Input: dimensioned drawing with shaded views. Units: mm. Origin: part minimum x, y, z. Give positions to 0.01 mm unless a question says otherwise; leave off trailing zeros. Order: outer loops, then holes, each group sorted by start corner. A loop starts at its lowest first (then second) coordinate and runs counter-clockwise, first axis right, second up. Notation, with made-up numbers: (35, 43.25) -> (43, 43.25) arc R35 ccw to (43, 80.25) -> close; hole circle Ø6 at (48, 19.25). An arc over 180 degrees is marked (long way). Use CSV: the item, a comma, the result in double quotes.
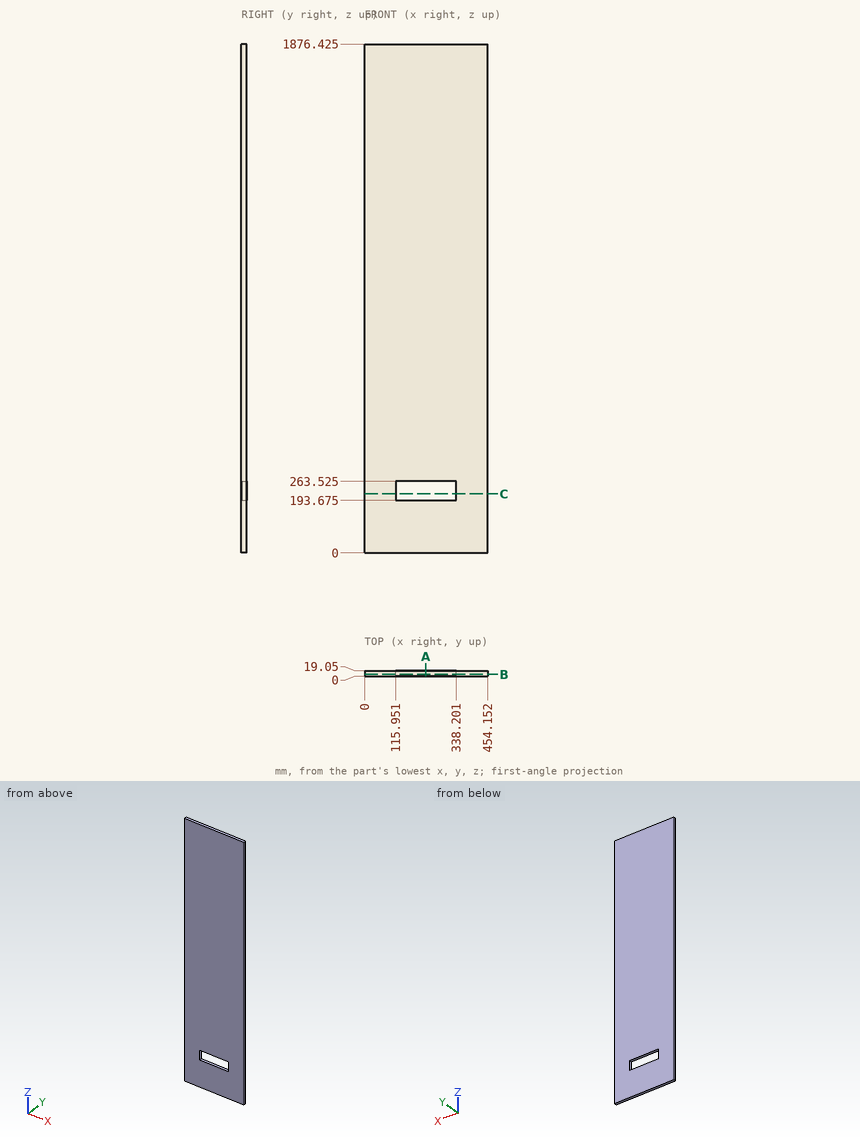
1. Section query A-A on x = 226.5. Return loops of the section in (y, z) (3 decimals), plus the area to 3 significant figures.
Answer below:
outline,"(0, 0) -> (19.05, 0) -> (19.05, 193.675) -> (0, 193.675) -> close; (0, 263.525) -> (19.05, 263.525) -> (19.05, 1876.425) -> (0, 1876.425) -> close"
area,"34,400 mm²"
2. Section query B-B on y = 6. Return loops of the section in (x, z) (3 decimals).
Answer below:
outline,"(0, 0) -> (454.152, 0) -> (454.152, 1876.425) -> (0, 1876.425) -> close; hole (115.951, 193.675) -> (338.201, 193.675) -> (338.201, 263.525) -> (115.951, 263.525) -> close"
3. Ray query, line 1 along Z through (x, y) = (288, 9) (3 decimals). Return the intervals inside material, ascending.
Answer below:
line 1,"z = 0 to 193.675, 263.525 to 1876.425"
4. Section query C-C on z = 217. Return loops of the section in (x, y), plus the area to 3 significant figures.
Answer below:
outline,"(0, 0) -> (115.95, 0) -> (115.95, 19.05) -> (0, 19.05) -> close; (338.2, 0) -> (454.15, 0) -> (454.15, 19.05) -> (338.2, 19.05) -> close"
area,"4,420 mm²"
